from build123d import *

# Parameters (mm, degrees)
F0_R     = 19.05
F1_DEPTH = 6.35
F2_R     = 6.34999


# Not quite as in the source:
# - a fillet or chamfer is up to 0.001 mm smaller than in the source, because OpenCascade refuses the exact size


with BuildPart() as f1:
    # F0 (on Right) → F1 (new body, symmetric)
    with BuildSketch(Plane.YZ):
        Polygon((406.4, 0), (0, 0), (0, -101.6), (406.4, -203.2), align=None)
        with Locations((101.6, -76.2)):
            Circle(F0_R, mode=Mode.SUBTRACT)
    extrude(amount=F1_DEPTH, both=True)

    # F2 (radius 6.35 in the source; OpenCascade refuses exactly that, so slightly less here)
    f2_edges = [f1.edges().sort_by_distance(p)[0] for p in [
        (-6.35, 203.2, -152.4),
        (6.35, 203.2, -152.4),
        (6.35, 0, -50.8),
        (-6.35, 0, -50.8),
    ]]
    fillet(f2_edges, radius=F2_R)


solid = f1.part
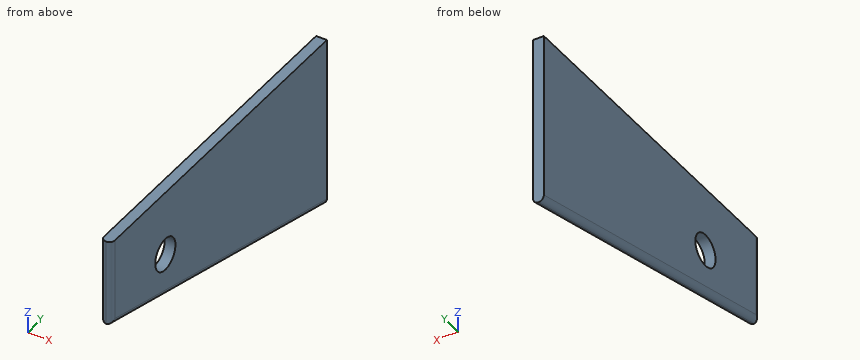
Geometry check sheet. Reference: the model listing, model coordinates, mm. Give positions to 0.01 mm unless a question says otherwise; leave off trailing zeros. Write each loop counter-clockwise with the first axis right and the second up, starting at its lowest first coordinate (ties: lowest second). Pieces come first, ordered by that corner, then holes. Notation, with made-up numbers: M -23.75,34 L 20.25,34 A23 cw 20.25,68 Z; hole C 2.25,-27 d3. An arc over 180 degrees is marked long. Answer as CSV lines item,"result". Start each with the question number.
Q1. Go/stop test with flat-tipped pins: pin 1 (4 mm diameter, centred on x = -4, y = 320, fed in from -Z); pin 2 (5 mm diameter, centred on y = 155.5, z = -139, fed in from -X); pin 3 (8 mm diameter, centred on y = 94, z = -127.5, fed in from -X). Record where each tip stops, or that it passes through.
Q2. Material ranges on L1, parallel to Z at x = -1.5, y = 101.6; L2, parallel to Z at x = 2.5, y = 101.6; L3, parallel to Y at x = -2.5, z = -90, recorded low to high.
Q3. Section check B-B, the plane x = 3.5. Record the cut outline in (y, z).
Geometry says:
1,pin 1,"z = -181.42"
1,pin 2,"x = -5.87"
1,pin 3,"x = -4.29"
2,L1,"-126.81 to -95.25, -57.15 to 0"
2,L2,"-126.47 to -95.25, -57.15 to 0"
2,L3,"0.51 to 88.47, 114.73 to 406.4"
3,outline,"M 1.05,-100.78 L 406.4,-202.12 L 406.4,0 L 1.05,0 Z; hole C 101.6,-76.2 d38.1"
